```python
from build123d import *

# Parameters (mm, degrees)
EXTRUDE_1_DEPTH           = 545
FILLET_1_R                = 1
FILLET_2_R                = 1.95
CUT_EXTRUDE_START         = -31.8
CUT_EXTRUDE_1_OUTLINE_R   = 2.65
CUT_EXTRUDE_1_OUTLINE_R_2 = 5
CUT_EXTRUDE_1_DEPTH       = 23.6


# Read off the part's stored shape, not the designer's step: the extrude step
with BuildPart() as part:
    # Sketch 2 → Extrude 1 (new body)
    with BuildSketch(Plane.XY):
        Polygon((-29.99112912, -4.35), (-29.99112912, -19), (-29.99112912, -20), (-29, -20), (-6.74112912, -20), (-6.74112912, -19), (-6.74112912, -11.8), (6.74112912, -11.8), (6.74112912, -19), (6.74112912, -20), (29, -20), (29.99112912, -20), (29.99112912, -19), (29.99112912, -4.35), (29.05, -4.35), (29.042967642, -6.1), (21.81774176, -6.1), (21.81774176, 6.1), (29.042967642, 6.1), (29.05, 4.35), (29.99112912, 4.35), (29.99112912, 19), (29.99112912, 20), (29, 20), (6.74112912, 20), (6.74112912, 19), (6.74112912, 11.8), (0.00887088, 11.8), (-6.74112912, 11.8), (-6.74112912, 19), (-6.74112912, 20), (-29, 20), (-29.99112912, 20), (-29.99112912, 19), (-29.99112912, 4.35), (-29.05, 4.35), (-29.042967642, 6.1), (-21.8, 6.1), (-21.8, -6.1), (-29.042967642, -6.1), (-29.05, -4.35), align=None)
        Polygon((-21.8, -7.3), (-21.8, -11.8), (-7.94112912, -11.8), (-7.94112912, -19), (-28.99112912, -19), (-29.038145454, -7.3), align=None, mode=Mode.SUBTRACT)
        Polygon((7.94112912, -11.8), (21.81774176, -11.8), (21.81774176, -7.3), (29.038145454, -7.3), (28.99112912, -19), (7.94112912, -19), align=None, mode=Mode.SUBTRACT)
        Polygon((-7.94112912, 11.8), (-21.8, 11.8), (-21.8, 7.3), (-29.038145454, 7.3), (-28.99112912, 19), (-7.94112912, 19), align=None, mode=Mode.SUBTRACT)
        Polygon((-20.8, 10.8), (0, 10.8), (20.8, 10.8), (20.8, -10.8), (-20.8, -10.8), align=None, mode=Mode.SUBTRACT)
        Polygon((21.81774176, 7.3), (21.81774176, 11.8), (7.94112912, 11.8), (7.94112912, 19), (28.99112912, 19), (29.038145454, 7.3), align=None, mode=Mode.SUBTRACT)
    extrude(amount=EXTRUDE_1_DEPTH)

    # Fillet 1
    fillet_1_edges = [part.edges().sort_by_distance(p)[0] for p in [
        (29.99112912, 20, 272.5),
        (29.99112912, -20, 272.5),
        (-29.99112912, -20, 272.5),
        (-29.99112912, 20, 272.5),
    ]]
    fillet(fillet_1_edges, radius=FILLET_1_R)

    # Fillet 2
    fillet_2_edges = [part.edges().sort_by_distance(p)[0] for p in [
        (-21.8, 11.8, 272.5),
        (21.81774176, -11.8, 272.5),
        (21.81774176, 11.8, 272.5),
        (-21.8, -11.8, 272.5),
    ]]
    fillet(fillet_2_edges, radius=FILLET_2_R)

    # Cut-Extrude 1 outline → Cut-Extrude 1 (cut)
    with BuildSketch(Plane(origin=(0, 20, 0), x_dir=(1, 0, 0), z_dir=(0, 1, 0)).offset(CUT_EXTRUDE_START)):
        with Locations((0, -30)):
            Circle(CUT_EXTRUDE_1_OUTLINE_R)
        with Locations((0, -375)):
            Circle(CUT_EXTRUDE_1_OUTLINE_R_2)
        with Locations((0, -455)):
            Circle(CUT_EXTRUDE_1_OUTLINE_R_2)
        with Locations((0, -535)):
            Circle(CUT_EXTRUDE_1_OUTLINE_R_2)
        with Locations((0, -10)):
            Circle(CUT_EXTRUDE_1_OUTLINE_R)
    extrude(amount=CUT_EXTRUDE_1_DEPTH, mode=Mode.SUBTRACT)


solid = part.part
```
Build history of the part. All positions in model axes, mm. A direction names the side the tool comes from. Give positions to 0.01 mm unless a question says otherwise; leave off trailing zeros.
1) Two-plate mould, pull along Z, no slides. Class faces 1 (the face through (-0.651, -11.307, 370.043)), 2 (the face through (-19, 19, 269)), 3 (the face through (-7, -12, 545)): released by +Z, released by -Z, zero draft, split by the parting line, or undercut.
Values follow:
face 1: undercut
face 2: zero draft
face 3: released by +Z
2) Probe line 1 along Y through (x, z) = (-20, 291); line 2 along Y through (x, z) = (26.5, 189.5); line 3 along X through (y, z) = (-14, 305). List the from-to ranges inside material, lowest first.
Values follow:
line 1: y = -20 to -19, -11.79 to -10.8, 10.8 to 11.79, 19 to 20
line 2: y = -20 to -19, -7.3 to -6.1, 6.1 to 7.3, 19 to 20
line 3: x = -29.99 to -29.01, -7.94 to -6.74, 6.74 to 7.94, 29.01 to 29.99
3) 3-axis set-ups, long thin cutter, end or side, ignore diameter. For faces 4 (the face through (0, 11.8, 269)), 5 (the face through (-18, 20, 269)), 6 (the face through (19, -19, 269)): which of +Z, -Z, +X, -X, +Y, -Y reach the whole face in a straight line?
Values follow:
face 4: +Z, -Z, +Y
face 5: +Z, -Z, +X, -X, +Y
face 6: +Z, -Z
4) Band-saw the part on A-A on z = 455. State how many separate pieces and enclosed holes the cut face has, then the cut area to 3 significant figures.
Values follow:
separate pieces: 2
enclosed holes: 4
area: 326 mm2
5) Drop flat-ended pins along their axis: P1, Ø7, axis at x = 0, z = 30, coming from the +Y side; P2, Ø13, axis at x = 0, z = 375, coming from the -Y side; P3, Ø0.5, axis at x = -29.5, z = 357, coming from the -Y side. Give the stop position or say it passes through.
Values follow:
P1: stops at y = 11.8
P2: stops at y = -11.8
P3: stops at y = -19.97
